Could you check a few things on this model? Use its own coordinates, in mm. Coordinates: 2 decimals unless noted, no trailing zeros. Loops run counter-clockwise (first coordinate to the right, second up) from the corner with the lowest first, then second, coordinate; pieces in that order, holes last. Notation, with made-up numbers: M -40,29 L 14,29 A12 cw 14,41 Z; hole C 87,2 d11. An arc over 180 degrees is marked long. Return JSON: item names as keys, results as strings. Group by question number.
from build123d import *

# Parameters (mm, degrees)
F0_W        = 10
F0_H        = 13
F1_DEPTH    = 7
F2_T1_DEPTH = 31.1932339785
F2_T3_DEPTH = 28.1932339785


# Not quite as in the source:
# - a fillet or chamfer that OpenCascade refuses, or shapes differently, is made with other operations: its cross-section is extruded or revolved along the edge and cut away or added
# - a feature of the source that left no trace in its solid (it failed there, or was rolled back) is left out


with BuildPart() as f1:
    # F0 (on Top) → F1 (new body)
    with BuildSketch(Plane.XY):
        Rectangle(F0_W, F0_H)
    extrude(amount=F1_DEPTH)

    # F2: chamfer of 0.5 x 3.5 on 8 edges, made by hand

    # F2_s2 → F2_t1 (cut)
    with BuildSketch(Plane.XZ.offset(-15.5966169892)):
        Polygon((-5, 3.5), (-4.5, 7), (-5, 7), align=None)
        Polygon((5, 3.5), (4.5, 7), (5, 7), align=None)
        Polygon((-5, 3.5), (-4.5, 0), (-5, 0), align=None)
        Polygon((5, 3.5), (4.5, 0), (5, 0), align=None)
    extrude(amount=F2_T1_DEPTH, mode=Mode.SUBTRACT)

    # F2_s4 → F2_t3 (cut)
    with BuildSketch(Plane.YZ.offset(-14.0966169892)):
        Polygon((-6.5, 3.5), (-6, 7), (-6.5, 7), align=None)
        Polygon((6.5, 3.5), (6, 7), (6.5, 7), align=None)
        Polygon((-6.5, 3.5), (-6, 0), (-6.5, 0), align=None)
        Polygon((6.5, 3.5), (6, 0), (6.5, 0), align=None)
    extrude(amount=F2_T3_DEPTH, mode=Mode.SUBTRACT)


solid = f1.part
(1) Imagine slicing it at C-C, the plane z = 4.5. Write out the boundary of the cut face in (x, y).
(2) Imagine slicing it at D-D, the plane z = 2.75. Write out the boundary of the cut face in (x, y).
(3) If I drill on L1, parallel to X at y = -2.5, z = 3.75; L2, parallel to X at y = -6, z = 5; L3, parallel to Y at x = -2.5, z = 1.5, over which ranges is the centre line in solid material (lowest first)? Write a range as [from, to].
(4) Will these pins go through, and if not, where does the flat tip stop? P1, Ø3, axis at y = 0.5, z = 1.5, coming from the +X side; P2, Ø1.5, axis at x = -0.5, y = 2.5, coming from the -Z side.
(5) Imagine slicing it at A-A, the plane x = 0. Write out the boundary of the cut face in (y, z).
(6) Imagine slicing it at B-B, the plane y = -4.5. Write out the boundary of the cut face in (x, z), then the cut area to 3 significant figures.
Checks:
{
 "1": {"outline": "M -4.86,-6.36 L 4.86,-6.36 L 4.86,6.36 L -4.86,6.36 Z"},
 "2": {"outline": "M -4.89,-6.39 L 4.89,-6.39 L 4.89,6.39 L -4.89,6.39 Z"},
 "3": {"L1": "[-4.96, 4.96]", "L2": "[-4.79, 4.79]", "L3": "[-6.21, 6.21]"},
 "4": {"P1": "x = 4.93", "P2": "z = 0"},
 "5": {"outline": "M -6.5,3.5 L -6,0 L 6,0 L 6.5,3.5 L 6,7 L -6,7 Z"},
 "6": {"outline": "M -5,3.5 L -4.5,0 L 4.5,0 L 5,3.5 L 4.5,7 L -4.5,7 Z", "area": "66.5 mm²"}
}
